from build123d import *

# Parameters (mm, degrees)
F0_R      = 3.475
F1_DEPTH  = 3.85
F2_R      = 2.425
F3_DEPTH  = 2
F5_DEPTH  = 1
F6_R      = 2.325
F7_DEPTH  = 1
F8_R      = 1.275
F9_DEPTH  = 2.851
F10_R     = 0.5
F11_DEPTH = 3.851


with BuildPart() as f1:
    # F0 (on Top) → F1 (new body)
    with BuildSketch(Plane.XY):
        Circle(F0_R)
    extrude(amount=F1_DEPTH)

    # F2 (on face) → F3 (cut)
    with BuildSketch(Plane(origin=(0, 0, 0), x_dir=(1, 0, 0), z_dir=(0, 0, -1))):
        Circle(F2_R)
    extrude(amount=-F3_DEPTH, mode=Mode.SUBTRACT)

    # F4 (on face) → F5 (join)
    with BuildSketch(Plane.XY.offset(3.85)):
        with BuildLine():
            Line((14.22, 2), (0, 3.475))
            ThreePointArc((0, 3.475), (-3.475, 0), (0, -3.475))
            Line((0, -3.475), (14.22, -2))
            ThreePointArc((14.22, -2), (16.023276, 0), (14.22, 2))
        make_face()
    extrude(amount=-F5_DEPTH)

    # F6 (on face) → F7 (cut)
    with BuildSketch(Plane.XY.offset(3.85)):
        Circle(F6_R)
    extrude(amount=-F7_DEPTH, mode=Mode.SUBTRACT)

    # F8 (on face) → F9 (cut, through all)
    with BuildSketch(Plane.XY.offset(2.85)):
        Circle(F8_R)
    extrude(amount=-F9_DEPTH, mode=Mode.SUBTRACT)

    # F10 (on face) → F11 (cut, through all)
    with BuildSketch(Plane.XY.offset(3.85)):
        with Locations((14.012546, 0)):
            Circle(F10_R)
        with Locations((12.042546, 0)):
            Circle(F10_R)
        with Locations((10.072546, 0)):
            Circle(F10_R)
        with Locations((8.102546, 0)):
            Circle(F10_R)
        with Locations((6.132546, 0)):
            Circle(F10_R)
        with Locations((4.162546, 0)):
            Circle(F10_R)
    extrude(amount=-F11_DEPTH, mode=Mode.SUBTRACT)

    # F12: F1 across plane


with BuildPart() as f1_1:
    add(f1.part)
    add(f1.part.mirror(Plane.YZ))


solid = f1_1.part
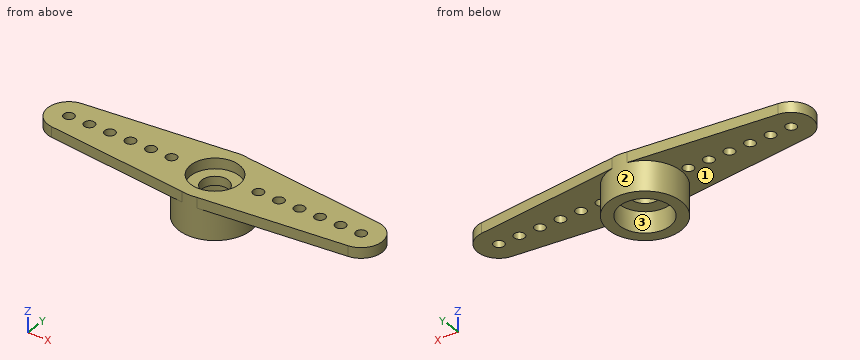
Can you work these out from the model? Positions are in its coordinate system, mm. Face numbers are marked on the shaded views. Give positions to 0.01 mm unless a question says otherwise; leave off trailing zeros. Loops run counter-clockwise (first coordinate to the right, second up) from the corner with the lowest first, then second, coordinate; pieces in that order, holes last. Notation, with made-up numbers: M 18.25,23.5 L 73.25,23.5 A11 cw 73.25,42.5 Z; hole C 14.25,-23 d5. An arc over 180 degrees is marked long. One line per item, written item: value. Start each with the question number.
1) If we section it at A-A, the plane x = 0: Write out the boundary of the cut face in (y, z) (3 decimals), and give its area (3 significant figures).
2) If we section it at D-D, the plane x = -10: Write out the boundary of the cut face in (y, z), and give its area (3 significant figures).
3) Thinking about a two-plate mould opening in Y: for the marked faces 1, 2 and 3, which applies, +Y half, -Y half, draft (parallel to the pull), parting line (faces both ways), or undercut?
4) If I drill on line 1 (X direction, y = 0, z = 2.6) (3 decimals); line 2 (Z direction, x = -3.5, y = -2.75), over which ranges is the centre line in solid material (lowest first)? Write a range as [from, to].
5) I'm going to push flat-ended pins straight in: pin 1 (3 mm diameter, centred on x = 0, y = 0, fed in from -Z); pin 2 (1 mm diameter, centred on x = 3.5, z = 2, fed in from +Y). Where does each tip first touch, or does it pass through?
6) If we section it at C-C, the plane y = 2.75: Write out the boundary of the cut face in (x, z).
7) If we section it at B-B, the plane y = 1: Write out the boundary of the cut face in (x, z).
Completed:
1. outline: M -3.475,0 L -2.425,0 L -2.425,2 L -1.275,2 L -1.275,2.85 L -2.325,2.85 L -2.325,3.85 L -3.475,3.85 Z; M 1.275,2 L 2.425,2 L 2.425,0 L 3.475,0 L 3.475,3.85 L 2.325,3.85 L 2.325,2.85 L 1.275,2.85 Z
1. area: 10.2 mm^2
2. outline: M -2.44,2.85 L -0.49,2.85 L -0.49,3.85 L -2.44,3.85 Z; M 0.49,2.85 L 2.44,2.85 L 2.44,3.85 L 0.49,3.85 Z
2. area: 3.89 mm^2
3. face 1: draft
3. face 2: parting line
3. face 3: undercut
4. line 1: x = [-3.475, -1.275], [1.275, 3.475]
4. line 2: z = [2.85, 3.85]
5. pin 1: stops at z = 2
5. pin 2: stops at y = 1.75
6. outline: M -6.99,2.85 L -2.12,2.85 L -2.12,0 L 2.12,0 L 2.12,2.85 L 6.99,2.85 L 6.99,3.85 L -6.99,3.85 Z
7. outline: M -15.76,2.85 L -3.33,2.85 L -3.33,0 L -2.21,0 L -2.21,2 L -0.79,2 L -0.79,2.85 L -2.1,2.85 L -2.1,3.85 L -15.76,3.85 Z; M 0.79,2 L 2.21,2 L 2.21,0 L 3.33,0 L 3.33,2.85 L 15.76,2.85 L 15.76,3.85 L 2.1,3.85 L 2.1,2.85 L 0.79,2.85 Z
